Design review of the part built by this model. Coordinates are the model's own, in mm. A direction names the side the tool comes from. Round coordinates to 2 decimals unless told otherwise and drop trailing zeros. Write each loop counter-clockwise with the first axis right and the second up, starting at its lowest first coordinate (ties: lowest second). Pieces come first, ordered by that corner, then holes. Notation, with made-up numbers: (84, -21) -> (90, -21) arc R14 ccw to (90, -17) -> close; hole circle Ø6 at (67, -15). An arc over 180 degrees is marked (long way). Write item = value, one per line. Start each with the question number.
Item 1: For pin 1 Ø8 at (y, z) = (8, -1.5) entering from -X; pin 2 Ø5 at (y, z) = (6, -1) entering from +X; pin 3 Ø2 at (x, z) = (12.5, -15) entering from -Y (3 decimals), all flat-tipped, find the tip position at first contact; note any pin that passes through.
Item 2: Add section D-D, the plane y = 19.75. State the section outline as (x, z) points.
Item 3: Mouldability with a two-part tool opening along X and no side actions: class faces 3 (the flat face through (19, 15.748, -9)), 4 (the flat face through (20, 22.86, 5)), 5 (the cylindrical face through (13.91, 11.02, 18.14)) as released by +X, released by -X, zero draft, split by the parting line, or undercut.
Item 4: To check wall thickness, follow L1, parallel to X at y = 1.45, z = 0; L2, parallel to X at y = 20.75, z = 0; L3, parallel to Z at x = -1.5, y = 14.5. State the ranges of each line that lie inside material, in increasing order.
Item 5: Add section B-B, the plane x = 0. State the section outline as (y, z) points (3 decimals), then the cut area to 3 significant figures.
Item 6: Machinability: for faces 1 (the flat face through (14, 0, -17)), 2 (the cylindrical face through (18.929, 11.991, -9.845)), which of the approach directions +Z, -Z, +X, -X, +Y, -Y give a long, thin tool a straight path to every point of the face, cutting with its end or side? Answer none if there is none.
Item 7: Add section A-A, the plane z = 0. State the section outline as (x, y) points (3 decimals).
Item 8: Add section C-C, the plane y = 6.5. State the section outline as (x, z) points.
from build123d import *

# Parameters (mm, degrees)
CHAMFER1_SIZE       = 0.508
CHAMFER2_SIZE       = 0.254
BOSS_EXTRUDE1_REACH = 41.595
SKETCH2_R           = 22.86
SKETCH2_R_2         = 21.59


with BuildPart() as part:
    # Sketch1 → Revolve1 (revolve)
    with BuildSketch(Plane.XY, mode=Mode.PRIVATE) as revolve1_sk:
        Polygon((20.32, 22.225), (20.32, 22.86), (22.86, 22.86), (22.86, 0), (22.225, 0), (22.225, 2.413), (21.59, 2.413), (21.59, 5.588), (21.59, 8.128), (21.336, 8.128), (21.336, 15.748), (20.828, 15.748), (20.828, 21.59), (20.828, 22.225), align=None)
    revolve(revolve1_sk.sketch.rotate(Axis((0, -7.741318897, 0), (0, 1, 0)), 90), axis=Axis((0, -7.741318897, 0), (0, 1, 0)))

    # Chamfer1
    chamfer1_edges = [part.edges().sort_by_distance(p)[0] for p in [
        (0, 22.86, 22.86),
    ]]
    chamfer(chamfer1_edges, length=CHAMFER1_SIZE)

    # Chamfer2
    chamfer2_edges = [part.edges().sort_by_distance(p)[0] for p in [
        (0, 0, 22.225),
    ]]
    chamfer(chamfer2_edges, length=CHAMFER2_SIZE)

    # Sketch2 → Boss-Extrude1 (add, up to next)
    with BuildSketch(Plane.XZ, mode=Mode.PRIVATE) as boss_extrude1_sk1:
        with Locations(Location((0, 0, 0), (0, 0, 270))):
            Circle(SKETCH2_R)
        with Locations(Location((0, 0, 0), (0, 0, 270))):
            Circle(SKETCH2_R_2, mode=Mode.SUBTRACT)
    boss_extrude1_tool1 = extrude(boss_extrude1_sk1.sketch, amount=-BOSS_EXTRUDE1_REACH, mode=Mode.PRIVATE) - part.part
    add(boss_extrude1_tool1.solids().sort_by_distance((0, 0, 22.213422))[0])


solid = part.part
Result set:
q1.pin_1 = -22.86
q1.pin_2 = 22.86
q1.pin_3 = 22.225
q2.outline = circle Ø45.72 at (0, 0); hole circle Ø41.66 at (0, 0)
q3.face_3 = undercut
q3.face_4 = zero draft
q3.face_5 = split by the parting line
q4.L1 = -22.86 to -21.59, 21.59 to 22.86
q4.L2 = -22.86 to -20.83, 20.83 to 22.86
q4.L3 = -22.81 to -21.28, 21.28 to 22.81
q5.outline = (0, -22.86) -> (22.352, -22.86) -> (22.86, -22.352) -> (22.86, -20.32) -> (22.225, -20.32) -> (22.225, -20.828) -> (15.748, -20.828) -> (15.748, -21.336) -> (8.128, -21.336) -> (8.128, -21.59) -> (0, -21.59) -> close; (0, 21.59) -> (8.128, 21.59) -> (8.128, 21.336) -> (15.748, 21.336) -> (15.748, 20.828) -> (22.225, 20.828) -> (22.225, 20.32) -> (22.86, 20.32) -> (22.86, 22.352) -> (22.352, 22.86) -> (0, 22.86) -> close
q5.area = 73.2 mm²
q6.face_1 = +Z, -Z, +X, -X, -Y
q6.face_2 = -Y
q7.outline = (-22.86, 0) -> (-21.59, 0) -> (-21.59, 8.128) -> (-21.336, 8.128) -> (-21.336, 15.748) -> (-20.828, 15.748) -> (-20.828, 22.225) -> (-20.32, 22.225) -> (-20.32, 22.86) -> (-22.352, 22.86) -> (-22.86, 22.352) -> close; (20.32, 22.225) -> (20.828, 22.225) -> (20.828, 15.748) -> (21.336, 15.748) -> (21.336, 8.128) -> (21.59, 8.128) -> (21.59, 0) -> (22.86, 0) -> (22.86, 22.352) -> (22.352, 22.86) -> (20.32, 22.86) -> close
q8.outline = circle Ø45.72 at (0, 0); hole circle Ø43.18 at (0, 0)
